The model under review builds one solid part; all positions refer to its coordinate system, in mm. Coordinates: 2 decimals unless noted, no trailing zeros.
```python
from build123d import *

# Parameters (mm, degrees)
SKETCH1_W                   = 254
SKETCH1_H                   = 114.3
BOSS_EXTRUDE1_DEPTH         = 9.525
M3_CLEARANCE_HOLE1_D        = 4.45
M3_CLEARANCE_HOLE1_DEPTH    = 10
M3_CLEARANCE_HOLE1_TIP      = 1.336914877
F_3_8_CLEARANCE_HOLE1_D     = 9.8044
F_3_8_CLEARANCE_HOLE1_DEPTH = 10
F_3_8_CLEARANCE_HOLE1_TIP   = 2.945538927
M3_CLEARANCE_HOLE2_D        = 4.45
M3_CLEARANCE_HOLE2_DEPTH    = 10
M3_CLEARANCE_HOLE2_TIP      = 1.336914877
FILLET1_R                   = 2
M3_CLEARANCE_HOLE4_D        = 4.45
M3_CLEARANCE_HOLE4_DEPTH    = 10
M3_CLEARANCE_HOLE4_TIP      = 1.336914877
SKETCH18_R                  = 8
CUT_EXTRUDE1_DEPTH          = 140.5917194


with BuildPart() as part:
    # Sketch1 → Boss-Extrude1 (new body)
    with BuildSketch(Plane(origin=(0, 0, 0), x_dir=(1, 0, 0), z_dir=(0, 1, 0))):
        Rectangle(SKETCH1_W, SKETCH1_H)
    extrude(amount=BOSS_EXTRUDE1_DEPTH)

    # M3 Clearance Hole1
    with Locations(Plane(origin=(0, 9.525, 0), x_dir=(1, 0, 0), z_dir=(0, 1, 0))):
        with Locations((-80.5625, -15.621), (-80.5625, 15.621), (-118.6625, -15.621), (-118.6625, 15.621), (118.6625, -15.621), (80.5625, -15.621), (80.5625, 15.621), (118.6625, 15.621)):
            Hole(M3_CLEARANCE_HOLE1_D / 2, depth=M3_CLEARANCE_HOLE1_DEPTH)
            with Locations((0, 0, -(M3_CLEARANCE_HOLE1_DEPTH + M3_CLEARANCE_HOLE1_TIP / 2))):  # 118° drill point
                Cone(0, M3_CLEARANCE_HOLE1_D / 2, M3_CLEARANCE_HOLE1_TIP, mode=Mode.SUBTRACT)

    # 3/8 Clearance Hole1
    with Locations(Plane(origin=(0, 0, 0), x_dir=(-1, 0, 0), z_dir=(0, -1, 0))):
        with Locations((-112.7125, 42.8625), (-112.7125, -42.8625), (112.7125, -42.8625), (112.7125, 42.8625)):
            Hole(F_3_8_CLEARANCE_HOLE1_D / 2, depth=F_3_8_CLEARANCE_HOLE1_DEPTH)
            with Locations((0, 0, -(F_3_8_CLEARANCE_HOLE1_DEPTH + F_3_8_CLEARANCE_HOLE1_TIP / 2))):  # 118° drill point
                Cone(0, F_3_8_CLEARANCE_HOLE1_D / 2, F_3_8_CLEARANCE_HOLE1_TIP, mode=Mode.SUBTRACT)

    # M3 Clearance Hole2
    with Locations(Plane.XZ):
        with Locations((105, 20), (65, -20), (105, -20), (65, 20), (-65, -20), (-65, 20), (-105, 20), (-105, -20)):
            Hole(M3_CLEARANCE_HOLE2_D / 2, depth=M3_CLEARANCE_HOLE2_DEPTH)
            with Locations((0, 0, -(M3_CLEARANCE_HOLE2_DEPTH + M3_CLEARANCE_HOLE2_TIP / 2))):  # 118° drill point
                Cone(0, M3_CLEARANCE_HOLE2_D / 2, M3_CLEARANCE_HOLE2_TIP, mode=Mode.SUBTRACT)

    # Fillet1
    fillet1_edges = [part.edges().sort_by_distance(p)[0] for p in [
        (-127, 4.7625, -57.15),
        (127, 4.7625, -57.15),
        (127, 4.7625, 57.15),
        (-127, 4.7625, 57.15),
    ]]
    fillet(fillet1_edges, radius=FILLET1_R)

    # M3 Clearance Hole4
    with Locations(Plane.XZ):
        with Locations((0, -27), (-21.65, -0.55), (-37.55, -30.1), (37.55, 30.1), (21.65, 0.55), (0, 27)):
            Hole(M3_CLEARANCE_HOLE4_D / 2, depth=M3_CLEARANCE_HOLE4_DEPTH)
            with Locations((0, 0, -(M3_CLEARANCE_HOLE4_DEPTH + M3_CLEARANCE_HOLE4_TIP / 2))):  # 118° drill point
                Cone(0, M3_CLEARANCE_HOLE4_D / 2, M3_CLEARANCE_HOLE4_TIP, mode=Mode.SUBTRACT)

    # Sketch18 → Cut-Extrude1 (cut, through all)
    with BuildSketch(Plane.XZ):
        with Locations(Location((-51.75, 0, 0), (0, 0, 270))):
            Circle(SKETCH18_R)
        with Locations(Location((51.75, 0, 0), (0, 0, 270))):
            Circle(SKETCH18_R)
    extrude(amount=-CUT_EXTRUDE1_DEPTH, mode=Mode.SUBTRACT)


solid = part.part
```
(1) We need section A-A, the plane y = 2. Count the separate pieces of the cut face and the enclosed holes in it, and give its area (3 significant figures).
A:
separate pieces: 1
enclosed holes: 28
area: 28,000 mm2
(2) Draft analysis for pull direction Z (two halves, no side actions). For faces 1 (the face through (-106.196, 4.829, -18.124)), 2 (the face through (-2, 5, -57.15)), 3 (the face through (-2, 0, -1)), state which applies: released by +Z, released by -Z, zero draft, split by the parting line, or undercut.
A:
face 1: undercut
face 2: released by -Z
face 3: zero draft
(3) For pin 1 Ø3.5 at (x, z) = (-65, 20) entering from +Y, flat-tipped, find the tip position at first contact; note if it passes through.
A:
pin 1: passes through
(4) Wall thickness on probe 1 along Z at (x, y) = (-105, 3.75) (3 decimals); probe 2 along Z at (x, y) = (-112, 7.5); probe 3 along X at (y, z) = (5, 5) (3 decimals): over which ranges is each line inside the solid? List them lowest first.
A:
probe 1: z = -57.15 to -22.225, -17.775 to 17.775, 22.225 to 57.15
probe 2: z = -57.15 to -47.71, -38.01 to 38.01, 47.71 to 57.15
probe 3: x = -127 to -57.995, -45.505 to 45.505, 57.995 to 127
